CAD build for the part. Positions are in the model's coordinates, mm. Face numbers are marked on the shaded views. A direction names the side the tool comes from. Round coordinates to 2 decimals unless told otherwise and drop trailing zeros. Loops run counter-clockwise (first coordinate to the right, second up) from the corner with the lowest first, then second, coordinate; pieces in that order, holes last. Notation, with made-up numbers: M -32.75,8.5 L 19.25,8.5 A17 ccw 19.25,18.5 Z; hole C 42.5,7 d2. An arc over 180 degrees is marked long. One line per item, written item: value. Start each with the question number.
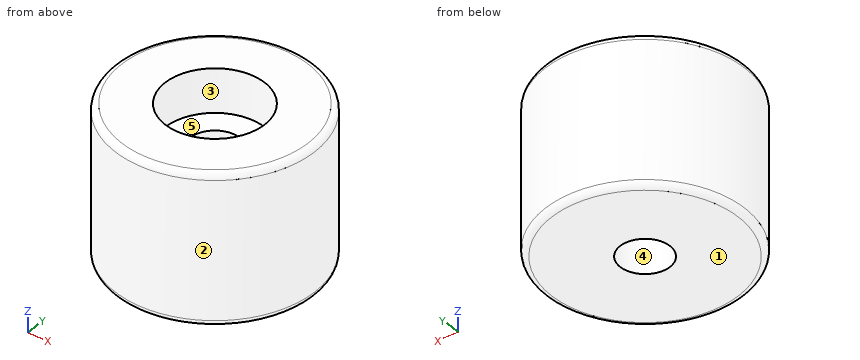
Autodesk Inventor part; units mm, degrees
ref_plane "YZ Plane" through (0, 0, 0) normal (1, 0, 0) x (0, 1, 0)
ref_plane "XZ Plane" through (0, 0, 0) normal (0, 1, 0) x (-1, 0, 0)
ref_plane "XY Plane" through (0, 0, 0) normal (0, 0, 1) x (1, 0, 0)
sketch "Sketch1" plane through (0, 0, 0) normal (0, 0, 1) x (1, 0, 0)
  circle A0 centre (0, 0) radius 8
  dimension "d0" = 16
extrude "Extrusion1" add sketch "Sketch1" along normal blind 12
sketch "Sketch2" plane through (0, 0, 12) normal (0, 0, 1) x (1, 0, 0)
  circle A0 centre (0, 0) radius 8
hole "Hole1" at (0, 0, 12) direction (0, 0, -1) diameter 4 end through all counterbore diameter 8 counterbore depth 3.5
fillet "Fillet1" radius 0.5 2 edges at (-8, 0, 12) (-8, 0, 0)
properties part number "Silicone Bed Spacers" material "Rubber, Silicone"
(1) Flat gauge pins, fed straight in: P1, Ø4, axis at x = 6.5, z = 2.5, coming from the +Y side; P2, Ø6, axis at x = 4.5, z = 4, coming from the +Y side; P3, Ø4, axis at x = -5, z = 4, coming from the +Y side. Where does each tip first touch, or does it go through?
(2) Slice it at C-C, the plane z = 2.5. List the corners of the cut face in (x, y).
(3) Mould opens along Y. For the marked faces 1, 2 and 3 say: pulls with the +Y half, pulls with the -Y half, needs draft (parallel to the pull), parting line crosses it, or undercut.
(4) Probe L1, parallel to Y at x = 0, z = 3; L2, parallel to Y at x = 0, z = 9.5; L3, parallel to Z at x = 3.75, y = 0.25. List the from-to ranges inside material, lowest first.
(5) Slice it at D-D, the plane z = 10.75. List the corners of the cut face in (x, y).
(6) Slice it at A-A, the plane x = 0. List the corners of the cut face in (y, z).
(7) Which spindle directions (+Z, -Z, +X, -X, +Y, -Y) get a long thin tool onto all of the face, cutting with end or side? Do the marked faces 4 and 5. Say none if no direction does.
Check result:
1. P1: stops at y = 6.61
1. P2: stops at y = 7.86
1. P3: stops at y = 7.42
2. outline: C 0,0 d16; hole C 0,0 d4
3. face 1: needs draft
3. face 2: parting line crosses it
3. face 3: undercut
4. L1: y = -8 to -2, 2 to 8
4. L2: y = -8 to -4, 4 to 8
4. L3: z = 0 to 8.5
5. outline: C 0,0 d16; hole C 0,0 d8
6. outline: M -8,0.5 A0.5 ccw -7.5,0 L -2,0 L -2,8.5 L -4,8.5 L -4,12 L -7.5,12 A0.5 ccw -8,11.5 Z; M 2,0 L 7.5,0 A0.5 ccw 8,0.5 L 8,11.5 A0.5 ccw 7.5,12 L 4,12 L 4,8.5 L 2,8.5 Z
7. face 4: +Z, -Z
7. face 5: +Z
